from build123d import *

# Parameters (mm, degrees)
SCHIZZO1_R                   = 147.5
SCHIZZO1_R_2                 = 90
ESTRUSIONE_ESTRUSIONE1_DEPTH = 12
TAGLIO_ESTRUSIONE1_DEPTH     = 8
SCHIZZO10_R                  = 3
TAGLIO_ESTRUSIONE2_DEPTH     = 4
RIPETIZIONECIRCOLARE3_COUNT  = 4


with BuildPart() as part:
    # Schizzo1 → Estrusione-Estrusione1 (new body)
    with BuildSketch(Plane.XY):
        Circle(SCHIZZO1_R)
        Circle(SCHIZZO1_R_2, mode=Mode.SUBTRACT)
    extrude(amount=ESTRUSIONE_ESTRUSIONE1_DEPTH)

    # Schizzo3 → Taglio-Estrusione1 (cut)
    with BuildSketch(Plane(origin=(0, 0, 0), x_dir=(-1, 0, 0), z_dir=(0, 0, -1))):
        with BuildLine():
            ThreePointArc((83.562389259, 99.585777605), (69.474068731, 98.353209271), (70.706637066, 84.264888743))
            ThreePointArc((70.706637066, 84.264888743), (67.682853372, -86.712348368), (-98.91169794, -48.12978299))
            ThreePointArc((-98.91169794, -48.12978299), (-112.279105297, -43.513245268), (-116.89564302, -56.880652625))
            ThreePointArc((-116.89564302, -56.880652625), (79.988826712, -102.478229889), (83.562389259, 99.585777605))
        make_face()
    extrude(amount=-TAGLIO_ESTRUSIONE1_DEPTH, mode=Mode.SUBTRACT)

    # Schizzo10 → Taglio-Estrusione2 (cut)
    with BuildSketch(Plane(origin=(0, 0, 8), x_dir=(-1, 0, 0), z_dir=(0, 0, -1))):
        with Locations((0, -120)):
            Circle(SCHIZZO10_R)
    extrude(amount=-TAGLIO_ESTRUSIONE2_DEPTH, mode=Mode.SUBTRACT)

    # Schizzo13 → Foro per Vite M6-1 (revolve, cut)
    with BuildSketch(Plane(origin=(-74.246212025, -74.246212025, 12), x_dir=(0, -1, 0), z_dir=(1, 0, 0))):
        Polygon((0, 0), (0, 7.922753981), (3.2, 6), (3.2, 0), align=None)
    foro_per_vite_m6_1 = revolve(axis=Axis((-74.246212025, -74.246212025, 18.35), (0, 0, -1)), mode=Mode.SUBTRACT)

    # RipetizioneCircolare3: Foro per Vite M6-1 ×4 about axis
    ripetizionecircolare3_axis = Axis((0, 0, 0), (0, 0, 1))
    for i in range(1, RIPETIZIONECIRCOLARE3_COUNT):
        add(foro_per_vite_m6_1.rotate(ripetizionecircolare3_axis, i * 360 / RIPETIZIONECIRCOLARE3_COUNT), mode=Mode.SUBTRACT)


solid = part.part
The listing builds one solid part. Answer for the finished solid, in the listing's coordinates (mm). A direction names the side the tool comes from. Round coordinates to 2 decimals unless told otherwise and drop trailing zeros. Order: outer loops, then holes, each group sorted by start corner. A loop starts at its lowest first (then second) coordinate and runs counter-clockwise, first axis right, second up. Notation, with made-up numbers: M -4.5,21 L 14.5,21 A15 ccw 14.5,45 Z; hole C 19,53.25 d1. An arc over 180 degrees is marked long. Answer in a Markdown table with one row per item. Add a question column.
1) The part is cut by section A-A on y = 0. Determine the outline of the cut face in (x, z), plus the area to 3 significant figures.
2) Which of the six approach directions +Z, -Z, +X, -X, +Y, -Y give full straight-line access (tool end or side, diameter ignored) to faces 1 (the face through (-75.723, 71.407, 9.042)), 2 (the face through (41.53, -79.845, 5.916)), 3 (the face through (-88, -74, 8))?
3) Flat-ended cylindrical pins translate along their axes: pin 1 Ø1.5 at (x, z) = (-77, 3) entering from -Y; pin 2 Ø1 at (y, z) = (43.5, 5) entering from +X; pin 3 Ø2 at (x, z) = (116, 6) entering from +Y. Find the tip coordinate at first contact, or state that the pin passes through.
4) The part is cut by section B-B on x = 42. Determine the outline of the cut face in (y, z), plus the area to 3 significant figures.
5) Consider line 1 along Y through (x, z) = (0, 6.5); line 2 along Y through (x, z) = (0, 9.15); line 3 along X through (y, z) = (5, 4.5). Determine where each line is inside the solid, lowest interval first. Write a range as from..to.
6) Determine the mould class of faces 4 (the face through (-31.98, -143.99, 5.92)), 5 (the face through (63, 68, 0)), 6 (the face through (-69.6, 98.5, 3.9)), 7 (the face through (-74.39, -71.05, 9.04)) for opening direction Y: pulls with the +Y half, pulls with the -Y half, needs draft (parallel to the pull), parting line crosses it, or undercut.
7) The part is cut by section C-C on y = -84.5. Determine the outline of the cut face in (x, z).
Findings below:
| question | item | result |
|---|---|---|
| 1 | outline | M -147.5,0 L -130,0 L -130,8 L -110,8 L -110,0 L -90,0 L -90,12 L -147.5,12 Z; M 90,0 L 147.5,0 L 147.5,12 L 90,12 Z |
| 1 | area | 1,220 mm² |
| 2 | face 1 | +Z |
| 2 | face 2 | +Z, -Z |
| 2 | face 3 | -Z |
| 3 | pin 1 | stops at y = -126.26 |
| 3 | pin 2 | stops at x = 141.09 |
| 3 | pin 3 | stops at y = 92.36 |
| 4 | outline | M -141.39,0 L -123.03,0 L -123.03,8 L -101.67,8 L -101.67,0 L -79.6,0 L -79.6,12 L -141.39,12 Z; M 79.6,0 L 141.39,0 L 141.39,12 L 79.6,12 Z |
| 4 | area | 1,310 mm² |
| 5 | line 1 | y = -147.5..-130, -110..-90, 90..147.5 |
| 5 | line 2 | y = -147.5..-123, -117..-90, 90..147.5 |
| 5 | line 3 | x = -147.42..-129.9, -109.89..-89.86, 89.86..147.42 |
| 6 | face 4 | parting line crosses it |
| 6 | face 5 | needs draft |
| 6 | face 6 | undercut |
| 6 | face 7 | undercut |
| 7 | outline | M -120.9,0 L -98.79,0 L -98.79,8 L -70.43,8 L -70.43,0 L -30.98,0 L -30.98,12 L -120.9,12 Z; M 30.98,0 L 70.43,0 L 70.43,8 L 98.79,8 L 98.79,0 L 120.9,0 L 120.9,12 L 30.98,12 Z |
